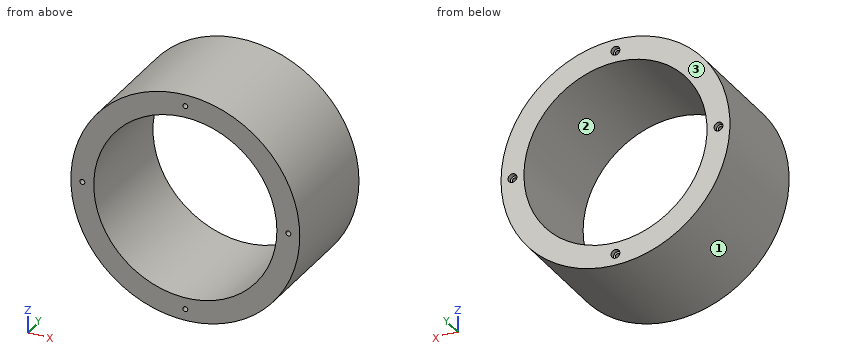
from build123d import *

# Parameters (mm, degrees)
F0_R            = 127
F0_R_2          = 101.6
F1_DEPTH        = 127
F3_D            = 5.5
F3_CBORE_D      = 9.75
F3_CBORE_DEPTH  = 5
F3_COPIES_COUNT = 4


# Not quite as in the source:
# - a pattern or mirror of a feature is missing from the dataset's text; its kind, count and spacing are read off the source's solid


with BuildPart() as f1:
    # F0 (on Front) → F1 (new body)
    with BuildSketch(Plane.XZ):
        Circle(F0_R)
        Circle(F0_R_2, mode=Mode.SUBTRACT)
    extrude(amount=F1_DEPTH)

    # F3 (through all)
    with Locations(Plane(origin=(0, 0, 0), x_dir=(-1, 0, 0), z_dir=(0, 1, 0))):
        with Locations((0, 0), (0, -114.3)):
            f3 = CounterBoreHole(F3_D / 2, F3_CBORE_D / 2, F3_CBORE_DEPTH)

    # F3_copies: F3 ×4 about axis
    f3_copies_axis = Axis((0, 0, 0), (0, 1, 0))
    for i in range(1, F3_COPIES_COUNT):
        add(f3.rotate(f3_copies_axis, i * 360 / F3_COPIES_COUNT), mode=Mode.SUBTRACT)


solid = f1.part
The listing builds one solid part. Answer for the finished solid, in the listing's coordinates (mm). Face numbers are marked on the shaded views. Coordinates: 2 decimals unless noted, no trailing zeros. Order: outer loops, then holes, each group sorted by start corner. A loop starts at its lowest first (then second) coordinate and runs counter-clockwise, first axis right, second up.
Q1. A cutting plane is placed at A-A, the plane x = -75. Write down the section's boundary in (y, z), and give its area (3 significant figures).
Q2. Consider line 1 (Z direction, x = 0, y = -2) (3 decimals); line 2 (Z direction, x = 0, y = -72); line 3 (X direction, y = -66.5, z = 35). Determine where each line is inside the solid, lowest interval first.
Q3. For a pull along X with two mould halves and no side action, classify the marked faces 1, 2 and 3 as pulls with the +X half, pulls with the -X half, needs draft (parallel to the pull), parting line crosses it, or undercut.
Q4. Given P1, Ø12, axis at x = 89, y = -17.5, coming from the -Z side; P2, Ø5, axis at y = -38.5, z = -65, coming from the +X side; P3, Ø10, axis at x = 83.5, y = -32, coming from the +Z side, each flat-ended and moving along its own axis, determine where each tip first touches the part or whether it passes through.
Q5. A cutting plane is placed at B-B, the plane z = -25. Write down the section's boundary in (x, y), and give its area (3 significant figures).
Q6. A cutting plane is placed at C-C, the plane y = -16. Write down the section's boundary in (x, z).
Answers follow:
1. outline: (-127, -102.49) - (0, -102.49) - (0, -68.54) - (-127, -68.54) - close; (-127, 68.54) - (0, 68.54) - (0, 102.49) - (-127, 102.49) - close
1. area: 8,620 mm2
2. line 1: z = -127 to -119.175, -109.425 to -101.6, 101.6 to 109.425, 119.175 to 127
2. line 2: z = -127 to -117.05, -111.55 to -101.6, 101.6 to 111.55, 117.05 to 127
2. line 3: x = -122.08 to -95.38, 95.38 to 122.08
3. face 1: parting line crosses it
3. face 2: undercut
3. face 3: needs draft
4. P1: stops at z = -96.12
4. P2: stops at x = 110.56
4. P3: stops at z = 99.83
5. outline: (-124.52, -127) - (-98.48, -127) - (-98.48, 0) - (-124.52, 0) - close; (98.48, -127) - (124.52, -127) - (124.52, 0) - (98.48, 0) - close
5. area: 6,610 mm2
6. outline: circle Ø254 at (0, 0); hole circle Ø5.5 at (-114.3, 0); hole circle Ø203.2 at (0, 0); hole circle Ø5.5 at (0, -114.3); hole circle Ø5.5 at (0, 114.3); hole circle Ø5.5 at (114.3, 0)
